Could you check a few things on this model? Use its own coordinates, in mm. A direction names the side the tool comes from. Give positions to 0.01 mm unless a question says otherwise; leave off trailing zeros. Write each loop counter-clockwise with the first axis right and the second up, starting at its lowest first coordinate (ties: lowest second). Pieces come first, ordered by that corner, then holes. Notation, with made-up numbers: M -13.75,54 L 0.25,54 A12 cw 0.25,63 Z; hole C 60,85.5 d5. An arc over 180 degrees is marked long. One line per item, written item: value.
```python
from build123d import *

# Parameters (mm, degrees)
F0_R     = 1.5
F0_R_2   = 5
F1_DEPTH = 12.5
F3_DEPTH = 5


with BuildPart() as f1:
    # F0 (on Top) → F1 (new body)
    with BuildSketch(Plane.XY):
        with BuildLine():
            ThreePointArc((18, 18), (17.414214, 19.414214), (16, 20))
            Line((16, 20), (-16, 20))
            ThreePointArc((-16, 20), (-17.414214, 19.414214), (-18, 18))
            Line((-18, 18), (-18, -18))
            ThreePointArc((-18, -18), (-17.414214, -19.414214), (-16, -20))
            Line((-16, -20), (16, -20))
            ThreePointArc((16, -20), (17.414214, -19.414214), (18, -18))
            Line((18, -18), (18, 18))
        make_face()
        with Locations((-9, 9)):
            Circle(F0_R, mode=Mode.SUBTRACT)
        Circle(F0_R_2, mode=Mode.SUBTRACT)
        with Locations((9, 9)):
            Circle(F0_R, mode=Mode.SUBTRACT)
    extrude(amount=F1_DEPTH)

    # F2 (on face) → F3 (join)
    with BuildSketch(Plane.XY.offset(12.5)):
        with BuildLine():
            Line((-18, 18), (-18, 15))
            Line((-18, 15), (18, 15))
            Line((18, 15), (18, 18))
            ThreePointArc((18, 18), (17.414214, 19.414214), (16, 20))
            Line((16, 20), (-16, 20))
            ThreePointArc((-16, 20), (-17.414214, 19.414214), (-18, 18))
        make_face()
        with BuildLine():
            Line((18, -15), (-18, -15))
            Line((-18, -15), (-18, -18))
            ThreePointArc((-18, -18), (-17.414214, -19.414214), (-16, -20))
            Line((-16, -20), (16, -20))
            ThreePointArc((16, -20), (17.414214, -19.414214), (18, -18))
            Line((18, -18), (18, -15))
        make_face()
    extrude(amount=F3_DEPTH)


solid = f1.part
```
1) I'm going to push flat-ended pins straight in: pin 1 (6 mm diameter, centred on x = 11.5, y = 9.5, fed in from +Z); pin 2 (2.5 mm diameter, centred on x = -9, y = 9, fed in from -Z). Where does each tip first touch, or does it pass through?
Outcome:
pin 1: stops at z = 12.5
pin 2: passes through
2) On a 3-axis mill with a long thin cutter (end or side, diameter ignored), from which of +Z, -Z, +X, -X, +Y, -Y can I reach the whole of each face in a straight line? I mean faces 1 (the face through (0, -15, 15)), 2 (the face through (0, -17, 17.5)). Say none if no direction works.
Outcome:
face 1: +Z, +X, -X
face 2: +Z, +X, -X, +Y, -Y
3) We'd pull the mould along X, two halves only. Please class faces 3 (the face through (18, 0, 7)), 4 (the face through (0, 18, 17.5)), 5 (the face through (7.8, 8.1, 6.2)), 6 (the face through (-1.08, -4.88, 6.16)): pulls with the +X half, pulls with the -X half, needs draft (parallel to the pull), parting line crosses it, or undercut.
Outcome:
face 3: pulls with the +X half
face 4: needs draft
face 5: undercut
face 6: undercut
4) If we section it at C-C, the plane z = 13: Write out the boundary of the cut face in (x, y).
Outcome:
outline: M -18,-18 A2 ccw -16,-20 L 16,-20 A2 ccw 18,-18 L 18,-15 L -18,-15 Z; M -18,15 L 18,15 L 18,18 A2 ccw 16,20 L -16,20 A2 ccw -18,18 Z
5) Please list where these lines run through material, in increasing order: L1, parallel to Y at x = 5, z = 14; L2, parallel to Y at x = 9, z = 7.75; L3, parallel to Z at x = -9, y = -7. Write a range as from..to.
Outcome:
L1: y = -20..-15, 15..20
L2: y = -20..7.5, 10.5..20
L3: z = 0..12.5
6) If we section it at B-B, the plane x = 9: Write out the boundary of the cut face in (y, z).
Outcome:
outline: M -20,0 L 7.5,0 L 7.5,12.5 L -15,12.5 L -15,17.5 L -20,17.5 Z; M 10.5,0 L 20,0 L 20,17.5 L 15,17.5 L 15,12.5 L 10.5,12.5 Z
7) If we section it at D-D, the plane y = 9: Write out the boundary of the cut face in (x, z), then the cut area to 3 significant figures.
Outcome:
outline: M -18,0 L -10.5,0 L -10.5,12.5 L -18,12.5 Z; M -7.5,0 L 7.5,0 L 7.5,12.5 L -7.5,12.5 Z; M 10.5,0 L 18,0 L 18,12.5 L 10.5,12.5 Z
area: 375 mm^2
8) If we section it at A-A, the plane y = 3: Write out the boundary of the cut face in (x, z), then the cut area to 3 significant figures.
Outcome:
outline: M -18,0 L -4,0 L -4,12.5 L -18,12.5 Z; M 4,0 L 18,0 L 18,12.5 L 4,12.5 Z
area: 350 mm^2
